Work out the finished part from the listing and answer in its coordinate system (mm). A direction names the side the tool comes from. Round coordinates to 2 decimals unless told otherwise and drop trailing zeros. Loops run counter-clockwise (first coordinate to the right, second up) from the corner with the lowest first, then second, coordinate; pieces in that order, holes last. Notation, with made-up numbers: (62.25, 89.25) - (98.25, 89.25) arc R15 cw to (98.25, 104.25) - close; hole circle Ø1 at (16.5, 32.5). An arc over 180 degrees is marked (long way). Return JSON: item names as keys, results as strings.
from build123d import *

# Parameters (mm, degrees)
SKETCH1_W           = 70
SKETCH1_H           = 50
BOSS_EXTRUDE1_DEPTH = 50
SKETCH2_R           = 5
CUT_EXTRUDE1_DEPTH  = 100.498743711
SKETCH3_R           = 15
BOSS_EXTRUDE2_DEPTH = 10
FILLET1_R           = 3
FILLET2_R           = 10


with BuildPart() as part:
    # Sketch1 → Boss-Extrude1 (new body)
    with BuildSketch(Plane.XY):
        with Locations((35, 25)):
            Rectangle(SKETCH1_W, SKETCH1_H)
    extrude(amount=BOSS_EXTRUDE1_DEPTH)

    # Sketch2 → Cut-Extrude1 (cut, through all)
    with BuildSketch(Plane(origin=(70, 0, 0), x_dir=(0, 0, -1), z_dir=(1, 0, 0))):
        with Locations((-25, 25)):
            Circle(SKETCH2_R)
    extrude(amount=-CUT_EXTRUDE1_DEPTH, mode=Mode.SUBTRACT)

    # Sketch3 → Boss-Extrude2 (add)
    with BuildSketch(Plane(origin=(0, 0, 0), x_dir=(-1, 0, 0), z_dir=(0, 0, -1))):
        with Locations((-35, 25)):
            Circle(SKETCH3_R)
    extrude(amount=BOSS_EXTRUDE2_DEPTH)

    # Sketch4 → Revolve1 (revolve)
    with BuildSketch(Plane(origin=(35, 0, 0), x_dir=(0, 0, -1), z_dir=(1, 0, 0)), mode=Mode.PRIVATE) as revolve1_sk:
        Polygon((10, 25), (10, 35), (25, 26), (25, 25), align=None)
    revolve(revolve1_sk.sketch.rotate(Axis((35, 25, -10), (0, 0, -1)), 90), axis=Axis((35, 25, -10), (0, 0, -1)))

    # Fillet1
    fillet1_edges = [part.edges().sort_by_distance(p)[0] for p in [
        (50, 25, -10),
    ]]
    fillet(fillet1_edges, radius=FILLET1_R)

    # Fillet2
    fillet2_edges = [part.edges().sort_by_distance(p)[0] for p in [
        (0, 50, 25),
        (70, 50, 25),
        (70, 0, 25),
        (0, 0, 25),
    ]]
    fillet(fillet2_edges, radius=FILLET2_R)


solid = part.part
1) A tool of negligible diameter and unlimited length cuts with its end or side. For faces 4 (the flat face through (35, 0, 25)), 5 (the flat face through (40, 34, -10)), from which of +Z, -Z, +X, -X, +Y, -Y can it reach the whole face along a straight path? Write none if from no direction.
Verdict:
{"face 4": "+Z, -Z, +X, -X, -Y", "face 5": "-Z"}
2) Section B-B (x = 35) is taken. Give the vertices of the cut face in (y, z), and give its area (3 significant figures).
Verdict:
{"outline": "(0, 0) - (10, 0) - (10, -7) arc R3 ccw to (13, -10) - (15, -10) - (24, -25) - (26, -25) - (35, -10) - (37, -10) arc R3 ccw to (40, -7) - (40, 0) - (50, 0) - (50, 50) - (0, 50) - close; hole circle Ø10 at (25, 25)", "area": "2,880 mm2"}
3) Determine the mould class of faces 1 (the cylindrical face through (35.49, 20.12, 26.08)), 2 (the flat face through (70, 25, 19)), 3 (the cylindrical face through (2.85, 3.01, 25.35)) for opening direction Y: pulls with the +Y half, pulls with the -Y half, needs draft (parallel to the pull), parting line crosses it, or undercut.
Verdict:
{"face 1": "undercut", "face 2": "needs draft", "face 3": "pulls with the -Y half"}
4) Section A-A (z = 22) is taken. Give the vertices of the cut face in (x, y), and give its area (3 significant figures).
Verdict:
{"outline": "(0, 10) arc R10 ccw to (10, 0) - (60, 0) arc R10 ccw to (70, 10) - (70, 21) - (0, 21) - close; (0, 29) - (70, 29) - (70, 40) arc R10 ccw to (60, 50) - (10, 50) arc R10 ccw to (0, 40) - close", "area": "2,850 mm2"}
5) A flat-ended cylindrical pin translates along its axis: pin 1 (3 mm diameter, centred on x = 15, y = 29.5, fed in from -Z). Find the tip coordinate at first contact, or state that the pin passes through.
Verdict:
{"pin 1": "stops at z = 0"}
6) Section C-C (y = 25) is taken. Give the vertices of the cut face in (x, z).
Verdict:
{"outline": "(0, 0) - (20, 0) - (20, -7) arc R3 ccw to (23, -10) - (25, -10) - (34, -25) - (36, -25) - (45, -10) - (47, -10) arc R3 ccw to (50, -7) - (50, 0) - (70, 0) - (70, 20) - (0, 20) - close; (0, 30) - (70, 30) - (70, 50) - (0, 50) - close"}
7) Find the intervals of material crossed by L1, parallel to Y at x = 30, z = 25; L2, parallel to Z at x = 40.5, y = 3; L3, parallel to Y at x = 8, z = 25, in increasing order.
Verdict:
{"L1": "y = 0 to 20, 30 to 50", "L2": "z = 0 to 50", "L3": "y = 0.2 to 20, 30 to 49.8"}
8) Section D-D (z = 44) is taken. Give the vertices of the cut face in (x, y).
Verdict:
{"outline": "(0, 10) arc R10 ccw to (10, 0) - (60, 0) arc R10 ccw to (70, 10) - (70, 40) arc R10 ccw to (60, 50) - (10, 50) arc R10 ccw to (0, 40) - close"}
